Verification items for the finished model (mm, model axes). A direction names the side the tool comes from. Coordinates: 2 decimals unless noted, no trailing zeros. Loops run counter-clockwise (first coordinate to the right, second up) from the corner with the lowest first, then second, coordinate; pieces in that order, holes last. Notation, with made-up numbers: (65.25, 15.25) - (100.25, 15.25) arc R15 cw to (100.25, 31.25) - close; hole circle Ø1 at (-21.75, 53). An arc over 180 degrees is marked (long way). Answer as CSV lines item,"result". Start each with the question number.
1. Cross-section at A-A (x = 67.5). Enter the section's corners in (y, z) (3 decimals), plus the area to 3 significant figures.
2. Set-up check for faces 1 (the flat face through (-3, -19.558, 0)), 2 (the flat face through (-3, -5.08, 22)): record each of +Z, -Z, +X, -X, +Y, -Y from which the full face is reachable in a straight line by a thin tool's end or side.
3. Material ranges on line 1 (Z direction, x = 203.2, y = -5.5) (3 decimals); line 2 (Y direction, x = -158, z = 22); line 3 (Z direction, x = -201.5, y = -15.5) (3 decimals), recorded low to high. Write a range as [from, to].
```python
from build123d import *

# Parameters (mm, degrees)
F0_W     = 457.2
F0_H     = 57.15
F1_DEPTH = 19.558
F2_W     = 5.08
F2_H     = 12.7
F3_DEPTH = 457.2
F4_R     = 2.54
F5_DEPTH = 19.558


with BuildPart() as f1:
    # F0 (on Front) → F1 (new body)
    with BuildSketch(Plane.XZ):
        Rectangle(F0_W, F0_H)
    extrude(amount=F1_DEPTH)

    # F2 (on face) → F3 (cut, through all)
    with BuildSketch(Plane(origin=(-228.6, 0, 0), x_dir=(0, -1, 0), z_dir=(-1, 0, 0))):
        with Locations((2.54, 22.225)):
            Rectangle(F2_W, F2_H)
    extrude(amount=-F3_DEPTH, mode=Mode.SUBTRACT)

    # F4 (on face) → F5 (cut, through all)
    with BuildSketch(Plane.XZ.offset(19.558)):
        with BuildLine():
            ThreePointArc((-2.54, -6.35), (-1.796051, -8.146051), (0, -8.89))
            Line((0, -8.89), (0, -6.35))
            Line((0, -6.35), (-2.54, -6.35))
        make_face()
        with Locations((-203.2, -6.35)):
            Circle(F4_R)
        with BuildLine():
            ThreePointArc((-104.14, -6.35), (-101.6, -8.89), (-99.06, -6.35))
            Line((-99.06, -6.35), (-101.6, -6.35))
            Line((-101.6, -6.35), (-104.14, -6.35))
        make_face()
        with BuildLine():
            Line((-101.6, -6.35), (-99.06, -6.35))
            ThreePointArc((-99.06, -6.35), (-101.6, -3.81), (-104.14, -6.35))
            Line((-104.14, -6.35), (-101.6, -6.35))
        make_face()
        with BuildLine():
            ThreePointArc((205.74, -6.35), (203.2, -3.81), (200.66, -6.35))
            ThreePointArc((200.66, -6.35), (203.2, -8.89), (205.74, -6.35))
        make_face()
        with BuildLine():
            ThreePointArc((104.14, -6.35), (101.6, -3.81), (99.06, -6.35))
            Line((99.06, -6.35), (101.6, -6.35))
            Line((101.6, -6.35), (104.14, -6.35))
        make_face()
        with BuildLine():
            Line((101.6, -6.35), (99.06, -6.35))
            ThreePointArc((99.06, -6.35), (101.6, -8.89), (104.14, -6.35))
            Line((104.14, -6.35), (101.6, -6.35))
        make_face()
        with BuildLine():
            Line((0, -6.35), (0, -8.89))
            ThreePointArc((0, -8.89), (1.796051, -8.146051), (2.54, -6.35))
            Line((2.54, -6.35), (0, -6.35))
        make_face()
        with BuildLine():
            Line((-2.54, -6.35), (0, -6.35))
            Line((0, -6.35), (2.54, -6.35))
            ThreePointArc((2.54, -6.35), (0, -3.81), (-2.54, -6.35))
        make_face()
    extrude(amount=-F5_DEPTH, mode=Mode.SUBTRACT)


solid = f1.part
```
Values follow:
1,outline,"(-19.558, -28.575) - (0, -28.575) - (0, 15.875) - (-5.08, 15.875) - (-5.08, 28.575) - (-19.558, 28.575) - close"
1,area,"1,050 mm²"
2,face 1,"+Z, -Z, +X, -X, -Y"
2,face 2,"+Z, +X, -X, +Y"
3,line 1,"z = [-28.575, -8.89], [-3.81, 28.575]"
3,line 2,"y = [-19.56, -5.08]"
3,line 3,"z = [-28.575, -8.237], [-4.463, 28.575]"
